```python
from build123d import *

# Parameters (mm, degrees)
F0_R     = 63.5
F0_R_2   = 9.525
F0_R_3   = 1.5875
F1_DEPTH = 4.7625


with BuildPart() as f1:
    # F0 (on Front) → F1 (new body)
    with BuildSketch(Plane.XZ):
        Circle(F0_R)
        with Locations((-25.4, -43.994091)):
            Circle(F0_R_2, mode=Mode.SUBTRACT)
        with Locations((-43.994091, -25.4)):
            Circle(F0_R_2, mode=Mode.SUBTRACT)
        with Locations((0, -50.8)):
            Circle(F0_R_2, mode=Mode.SUBTRACT)
        with Locations((25.4, -43.994091)):
            Circle(F0_R_2, mode=Mode.SUBTRACT)
        with Locations((43.994091, -25.4)):
            Circle(F0_R_2, mode=Mode.SUBTRACT)
        with Locations((-50.8, 0)):
            Circle(F0_R_2, mode=Mode.SUBTRACT)
        with Locations((-43.994091, 25.4)):
            Circle(F0_R_2, mode=Mode.SUBTRACT)
        with Locations((-25.4, 43.994091)):
            Circle(F0_R_2, mode=Mode.SUBTRACT)
        Circle(F0_R_3, mode=Mode.SUBTRACT)
        with Locations((50.8, 0)):
            Circle(F0_R_2, mode=Mode.SUBTRACT)
        with Locations((43.994091, 25.4)):
            Circle(F0_R_2, mode=Mode.SUBTRACT)
        with Locations((25.4, 43.994091)):
            Circle(F0_R_2, mode=Mode.SUBTRACT)
        with Locations((0, 50.8)):
            Circle(F0_R_2, mode=Mode.SUBTRACT)
    extrude(amount=F1_DEPTH)


solid = f1.part
```
Model file for the job. Use its own axes, mm. Give positions to 0.01 mm unless a question says otherwise; leave off trailing zeros. Loops run counter-clockwise (first coordinate to the right, second up) from the corner with the lowest first, then second, coordinate; pieces in that order, holes last. Notation, with made-up numbers: (36.5, 61) -> (60.5, 61) arc R10 cw to (60.5, 74) -> close; hole circle Ø3 at (89.25, 30.5). An arc over 180 degrees is marked (long way). Use CSV: the item, a comma, the result in double quotes. Start each with the question number.
1) Mould opens along X. For faces 1 (the cylindrical face through (-42, -2.35, -3.65)), 2 (the cylindrical face through (-0.34, -2.35, -1.55)), 3 (the cylindrical face through (-13.77, -2.35, -61.99)), 4 (the flat face through (-1, -4.762, -13)) say: released by +X, released by -X, zero draft, split by the parting line, or undercut.
2) Slice it at C-C on x = -25. Give the cut face in (y, z).
3) Slice it at A-A on x = 0. Give the cut face in (y, z) (1 decimal), plus the area to 3 significant figures.
4) Wall check: line 1 (Z direction, x = 0, y = -1.1) (1 decimal); line 2 (Z direction, x = 50, y = -2.3); line 3 (Z direction, x = -17.5, y = -3.1). Give the ranges that are in metal, low to high.
5) Slice it at D-D on z = 49. Give the cut face in (x, y), plus the area to 3 significant figures.
6) Slice it at B-B on z = 19. Give the cut face in (x, y).
7) Flat gauge pins, fed straight in: pin 1 Ø17 at (x, z) = (-43.99, 25.4) entering from +Y; pin 2 Ø1.5 at (y, z) = (-2, -47) entering from +X. Where does each tip first touch, or does it go through?
Computed values:
1,face 1,"undercut"
1,face 2,"undercut"
1,face 3,"split by the parting line"
1,face 4,"zero draft"
2,outline,"(-4.76, -58.37) -> (0, -58.37) -> (0, -53.51) -> (-4.76, -53.51) -> close; (-4.76, -34.48) -> (0, -34.48) -> (0, 34.48) -> (-4.76, 34.48) -> close; (-4.76, 53.51) -> (0, 53.51) -> (0, 58.37) -> (-4.76, 58.37) -> close"
3,outline,"(-4.8, -63.5) -> (0, -63.5) -> (0, -60.3) -> (-4.8, -60.3) -> close; (-4.8, -41.3) -> (0, -41.3) -> (0, -1.6) -> (-4.8, -1.6) -> close; (-4.8, 1.6) -> (0, 1.6) -> (0, 41.3) -> (-4.8, 41.3) -> close; (-4.8, 60.3) -> (0, 60.3) -> (0, 63.5) -> (-4.8, 63.5) -> close"
3,area,"408 mm^2"
4,line 1,"z = -63.5 to -60.3, -41.3 to -1.6, 1.6 to 41.3, 60.3 to 63.5"
4,line 2,"z = -39.14 to -32.79, -18.01 to -9.49, 9.49 to 18.01, 32.79 to 39.14"
4,line 3,"z = -61.04 to -49.32, -38.67 to 38.67, 49.32 to 61.04"
5,outline,"(-40.39, -4.76) -> (-33.5, -4.76) -> (-33.5, 0) -> (-40.39, 0) -> close; (-17.3, -4.76) -> (-9.35, -4.76) -> (-9.35, 0) -> (-17.3, 0) -> close; (9.35, -4.76) -> (17.3, -4.76) -> (17.3, 0) -> (9.35, 0) -> close; (33.5, -4.76) -> (40.39, -4.76) -> (40.39, 0) -> (33.5, 0) -> close"
5,area,"141 mm^2"
6,outline,"(-60.59, -4.76) -> (-51.05, -4.76) -> (-51.05, 0) -> (-60.59, 0) -> close; (-36.94, -4.76) -> (36.94, -4.76) -> (36.94, 0) -> (-36.94, 0) -> close; (51.05, -4.76) -> (60.59, -4.76) -> (60.59, 0) -> (51.05, 0) -> close"
7,pin 1,"passes through"
7,pin 2,"stops at x = 43.51"
